from build123d import *

# Parameters (mm, degrees)
SKETCH1_W           = 138
SKETCH1_H           = 170
BOSS_EXTRUDE1_DEPTH = 3
SKETCH2_R           = 2.1
SKETCH2_W           = 29
SKETCH2_H           = 30
CUT_EXTRUDE1_DEPTH  = 3
SKETCH3_R           = 2.1
SKETCH3_R_2         = 1.6
CUT_EXTRUDE2_DEPTH  = 219.981734398
FILLET1_R           = 10


with BuildPart() as part:
    # Sketch1 → Boss-Extrude1 (new body)
    with BuildSketch(Plane(origin=(0, 0, 0), x_dir=(1, 0, 0), z_dir=(0, 1, 0))):
        with Locations((69, 85)):
            Rectangle(SKETCH1_W, SKETCH1_H)
    extrude(amount=BOSS_EXTRUDE1_DEPTH)

    # Sketch2 → Cut-Extrude1 (cut)
    with BuildSketch(Plane(origin=(0, 3, 0), x_dir=(1, 0, 0), z_dir=(0, 1, 0))):
        with Locations(Location((69, 165, 0), (0, 0, 270))):
            Circle(SKETCH2_R)
        with Locations(Location((69, 5, 0), (0, 0, 270))):
            Circle(SKETCH2_R)
        with Locations((14.5, 155)):
            Rectangle(SKETCH2_W, SKETCH2_H)
        with Locations((123.5, 155)):
            Rectangle(SKETCH2_W, SKETCH2_H)
        with Locations((123.5, 15)):
            Rectangle(SKETCH2_W, SKETCH2_H)
        with Locations((14.5, 15)):
            Rectangle(SKETCH2_W, SKETCH2_H)
    extrude(amount=-CUT_EXTRUDE1_DEPTH, mode=Mode.SUBTRACT)

    # Sketch3 → Cut-Extrude2 (cut, through all)
    with BuildSketch(Plane(origin=(0, 3, 0), x_dir=(1, 0, 0), z_dir=(0, 1, 0))):
        with Locations(Location((14.25, 125, 0), (0, 0, 270))):
            Circle(SKETCH3_R)
        with Locations(Location((14.25, 45, 0), (0, 0, 270))):
            Circle(SKETCH3_R)
        with Locations(Location((14.25, 85, 0), (0, 0, 270))):
            Circle(SKETCH3_R)
        with Locations(Location((123.75, 45, 0), (0, 0, 90))):
            Circle(SKETCH3_R)
        with Locations(Location((123.75, 85, 0), (0, 0, 90))):
            Circle(SKETCH3_R)
        with Locations(Location((123.75, 125, 0), (0, 0, 90))):
            Circle(SKETCH3_R)
        with Locations(Location((8, 132, 0), (0, 0, 270))):
            Circle(SKETCH3_R_2)
        with Locations(Location((8, 38, 0), (0, 0, 270))):
            Circle(SKETCH3_R_2)
        with Locations(Location((130, 38, 0), (0, 0, 90))):
            Circle(SKETCH3_R_2)
        with Locations(Location((130, 132, 0), (0, 0, 90))):
            Circle(SKETCH3_R_2)
    extrude(amount=-CUT_EXTRUDE2_DEPTH, mode=Mode.SUBTRACT)

    # Fillet1
    fillet1_edges = [part.edges().sort_by_distance(p)[0] for p in [
        (138, 1.5, -140),
        (109, 1.5, -140),
        (109, 1.5, -170),
        (138, 1.5, -30),
        (109, 1.5, 0),
        (109, 1.5, -30),
        (0, 1.5, -30),
        (29, 1.5, -30),
        (29, 1.5, 0),
        (0, 1.5, -140),
        (29, 1.5, -170),
        (29, 1.5, -140),
    ]]
    fillet(fillet1_edges, radius=FILLET1_R)


solid = part.part
Work out the finished part from the listing and answer in its coordinate system (mm). Give positions to 0.01 mm unless a question says otherwise; leave off trailing zeros. Write each loop counter-clockwise with the first axis right and the second up, starting at its lowest first coordinate (ties: lowest second). Pieces come first, ordered by that corner, then holes.
Q1. Straight lines are drawn through the part: L1, parallel to Z at x = 14, y = 0.55; L2, parallel to X at y = 1.3, z = -133; L3, parallel to Z at x = 131, y = 1.05. For each, find the intervals that lie inside material, in ascending order.
Answer:
L1: z = -140 to -127.09, -122.91 to -87.09, -82.91 to -47.09, -42.91 to -30
L2: x = 0.46 to 6.75, 9.25 to 128.75, 131.25 to 137.54
L3: z = -139.54 to -133.25, -130.75 to -39.25, -36.75 to -30.46
Q2. For a pull along X with two mould halves and no side action, classify faces 1 (the face through (125.613, 1.521, -125.969)), 2 (the face through (2.85, 1.48, -136.99)), 3 (the face through (134.99, 1.48, -32.85)) as released by +X, released by -X, zero draft, split by the parting line, or undercut.
Answer:
face 1: undercut
face 2: released by -X
face 3: released by +X
Q3. The part is cut by section B-B on z = -45. Give the vertices of the cut face in (x, y), and give its area (3 significant figures).
Answer:
outline: (0, 0) - (12.15, 0) - (12.15, 3) - (0, 3) - close; (16.35, 0) - (121.65, 0) - (121.65, 3) - (16.35, 3) - close; (125.85, 0) - (138, 0) - (138, 3) - (125.85, 3) - close
area: 389 mm2
Q4. The part is cut by section C-C on y = 1.3. State how many separate pieces and enclosed holes the cut face has, and give its area (3 significant figures).
Answer:
separate pieces: 1
enclosed holes: 12
area: 19,800 mm2
Q5. The part is cut by section A-A on x = 69. Give the vertices of the cut face in (y, z).
Answer:
outline: (0, -170) - (3, -170) - (3, -167.1) - (0, -167.1) - close; (0, -162.9) - (3, -162.9) - (3, -7.1) - (0, -7.1) - close; (0, -2.9) - (3, -2.9) - (3, 0) - (0, 0) - close
Q6. The part is cut by section D-D on z = -16.5. Give the vertices of the cut face in (x, y).
Answer:
outline: (29, 0) - (109, 0) - (109, 3) - (29, 3) - close
Q7. Given pin 1 (5 mm diameter, centred on x = 69, z = -165, fed in from -Y); pin 2 (1.5 mm diameter, centred on y = 2, z = -154.5, fed in from +X); pin 3 (0.9 mm diameter, centred on x = 16, y = 1.5, fed in from +Z), each flat-ended and moving along its own axis, determine where each tip first touches the part or whether it passes through.
Answer:
pin 1: stops at y = 0
pin 2: stops at x = 109
pin 3: stops at z = -30
